from build123d import *

# Parameters (mm, degrees)
F1_DEPTH = 60
F2_SIZE  = 1


with BuildPart() as f1:
    # F0 (on Front) → F1 (new body)
    with BuildSketch(Plane.XZ):
        with BuildLine():
            Line((1.82927, 49.370132), (0, 50))
            Line((0, 50), (2.288286, 42.019797))
            ThreePointArc((2.288286, 42.019797), (1.404131, 39.441349), (-1.321078, 39.383352))
            Line((-1.321078, 39.383352), (-13.51647, 47.519061))
            Line((-13.51647, 47.519061), (-15.45085, 47.552826))
            Line((-15.45085, 47.552826), (-10.808542, 40.670321))
            ThreePointArc((-10.808542, 40.670321), (-10.852639, 37.944852), (-13.426545, 37.047558))
            Line((-13.426545, 37.047558), (-27.539125, 41.016494))
            Line((-27.539125, 41.016494), (-29.389263, 40.45085))
            Line((-29.389263, 40.45085), (-22.847355, 35.339751))
            ThreePointArc((-22.847355, 35.339751), (-22.047077, 32.734049), (-24.217728, 31.085291))
            Line((-24.217728, 31.085291), (-38.866057, 30.498946))
            Line((-38.866057, 30.498946), (-40.45085, 29.389263))
            Line((-40.45085, 29.389263), (-32.649709, 26.54988))
            ThreePointArc((-32.649709, 26.54988), (-31.083394, 24.319009), (-32.638311, 22.080179))
            Line((-32.638311, 22.080179), (-46.38851, 16.995949))
            Line((-46.38851, 16.995949), (-47.552826, 15.45085))
            Line((-47.552826, 15.45085), (-39.256083, 15.161121))
            ThreePointArc((-39.256083, 15.161121), (-37.077051, 13.523455), (-37.864029, 10.913705))
            Line((-37.864029, 10.913705), (-49.370132, 1.82927))
            Line((-49.370132, 1.82927), (-50, 0))
            Line((-50, 0), (-42.019797, 2.288286))
            ThreePointArc((-42.019797, 2.288286), (-39.441349, 1.404131), (-39.383352, -1.321078))
            Line((-39.383352, -1.321078), (-47.519061, -13.51647))
            Line((-47.519061, -13.51647), (-47.552826, -15.45085))
            Line((-47.552826, -15.45085), (-40.670321, -10.808542))
            ThreePointArc((-40.670321, -10.808542), (-37.944852, -10.852639), (-37.047558, -13.426545))
            Line((-37.047558, -13.426545), (-41.016494, -27.539125))
            Line((-41.016494, -27.539125), (-40.45085, -29.389263))
            Line((-40.45085, -29.389263), (-35.339751, -22.847355))
            ThreePointArc((-35.339751, -22.847355), (-32.734049, -22.047077), (-31.085291, -24.217728))
            Line((-31.085291, -24.217728), (-30.498946, -38.866057))
            Line((-30.498946, -38.866057), (-29.389263, -40.45085))
            Line((-29.389263, -40.45085), (-26.54988, -32.649709))
            ThreePointArc((-26.54988, -32.649709), (-24.319009, -31.083394), (-22.080179, -32.638311))
            Line((-22.080179, -32.638311), (-16.995949, -46.38851))
            Line((-16.995949, -46.38851), (-15.45085, -47.552826))
            Line((-15.45085, -47.552826), (-15.161121, -39.256083))
            ThreePointArc((-15.161121, -39.256083), (-13.523455, -37.077051), (-10.913705, -37.864029))
            Line((-10.913705, -37.864029), (-1.82927, -49.370132))
            Line((-1.82927, -49.370132), (0, -50))
            Line((0, -50), (-2.288286, -42.019797))
            ThreePointArc((-2.288286, -42.019797), (-1.404131, -39.441349), (1.321078, -39.383352))
            Line((1.321078, -39.383352), (13.51647, -47.519061))
            Line((13.51647, -47.519061), (15.45085, -47.552826))
            Line((15.45085, -47.552826), (10.808542, -40.670321))
            ThreePointArc((10.808542, -40.670321), (10.852639, -37.944852), (13.426545, -37.047558))
            Line((13.426545, -37.047558), (27.539125, -41.016494))
            Line((27.539125, -41.016494), (29.389263, -40.45085))
            Line((29.389263, -40.45085), (22.847355, -35.339751))
            ThreePointArc((22.847355, -35.339751), (22.047077, -32.734049), (24.217728, -31.085291))
            Line((24.217728, -31.085291), (38.866057, -30.498946))
            Line((38.866057, -30.498946), (40.45085, -29.389263))
            Line((40.45085, -29.389263), (32.649709, -26.54988))
            ThreePointArc((32.649709, -26.54988), (31.083394, -24.319009), (32.638311, -22.080179))
            Line((32.638311, -22.080179), (46.38851, -16.995949))
            Line((46.38851, -16.995949), (47.552826, -15.45085))
            Line((47.552826, -15.45085), (39.256083, -15.161121))
            ThreePointArc((39.256083, -15.161121), (37.077051, -13.523455), (37.864029, -10.913705))
            Line((37.864029, -10.913705), (49.370132, -1.82927))
            Line((49.370132, -1.82927), (50, 0))
            Line((50, 0), (42.019797, -2.288286))
            ThreePointArc((42.019797, -2.288286), (39.441349, -1.404131), (39.383352, 1.321078))
            Line((39.383352, 1.321078), (47.519061, 13.51647))
            Line((47.519061, 13.51647), (47.552826, 15.45085))
            Line((47.552826, 15.45085), (40.670321, 10.808542))
            ThreePointArc((40.670321, 10.808542), (37.944852, 10.852639), (37.047558, 13.426545))
            Line((37.047558, 13.426545), (41.016494, 27.539125))
            Line((41.016494, 27.539125), (40.45085, 29.389263))
            Line((40.45085, 29.389263), (35.339751, 22.847355))
            ThreePointArc((35.339751, 22.847355), (32.734049, 22.047077), (31.085291, 24.217728))
            Line((31.085291, 24.217728), (30.498946, 38.866057))
            Line((30.498946, 38.866057), (29.389263, 40.45085))
            Line((29.389263, 40.45085), (26.54988, 32.649709))
            ThreePointArc((26.54988, 32.649709), (24.319009, 31.083394), (22.080179, 32.638311))
            Line((22.080179, 32.638311), (16.995949, 46.38851))
            Line((16.995949, 46.38851), (15.45085, 47.552826))
            Line((15.45085, 47.552826), (15.161121, 39.256083))
            ThreePointArc((15.161121, 39.256083), (13.523455, 37.077051), (10.913705, 37.864029))
            Line((10.913705, 37.864029), (1.82927, 49.370132))
        make_face()
        with BuildLine():
            ThreePointArc((-4, -19.595918), (0, 20), (4, -19.595918))
            Line((4, -19.595918), (4, -23.595918))
            Line((4, -23.595918), (-4, -23.595918))
            Line((-4, -23.595918), (-4, -19.595918))
        make_face(mode=Mode.SUBTRACT)
    extrude(amount=F1_DEPTH)

    # F2
    f2_edges = [f1.edges().sort_by_distance(p)[0] for p in [
        (0, -60, 20),
        (0, 0, 20),
    ]]
    chamfer(f2_edges, length=F2_SIZE)


solid = f1.part
Work out the finished part from the listing and answer in its coordinate system (mm). A direction names the side the tool comes from. Coordinates: 2 decimals unless noted, no trailing zeros. Answer in a Markdown table with one row per item. Add a question column.
1. A tool of negligible diameter and unlimited length cuts with its end or side. For faces 1 (the flat face through (-31.439, -29.58, 30.796)), 2 (the flat face through (-4, -30, -22)), 3 (the flat face through (37.93, -29.58, 26.16)), 4 (the flat face through (26.16, -29.58, -37.93)), from which of +Z, -Z, +X, -X, +Y, -Y can it reach the whole face along a straight path? Write none if from no direction.
2. Flat-ended cylindrical pins translate along their axes: P1, Ø3, axis at x = -32, y = -36, coming from the +Z side; P2, Ø3, axis at x = -38.5, y = -41.5, coming from the -Z side; P3, Ø6, axis at y = -14.5, z = -0.5, coming from the -X side. Find the tip coordinate at first contact, or state that the pin passes through.
3. The mould has two halves that part along Z. Classify faces 5 (the flat face through (-39.004, -29.58, -20.384)), 6 (the cylindrical face through (13.56, -29.58, 37.09)), 7 (the flat face through (-1.128, -29.58, -46.066)), 8 (the cylindrical face through (-13.56, -29.58, -37.09)): pulls with the +Z half, pulls with the -Z half, needs draft (parallel to the pull), parting line crosses it, or undercut.
4. Consider L1, parallel to X at y = -31.5, z = -4.5; L2, parallel to Z at x = -6, y = -14; L3, parallel to Z at x = -7.5, y = -52.5. Determine where each line is inside the solid, lowest interval first.
Reported:
| question | item | result |
|---|---|---|
| 1 | face 1 | -X, +Y, -Y |
| 1 | face 2 | +Y, -Y |
| 1 | face 3 | +Z, +Y, -Y |
| 1 | face 4 | +X, +Y, -Y |
| 2 | P1 | stops at z = 30.83 |
| 2 | P2 | stops at z = -28.81 |
| 2 | P3 | stops at x = -50 |
| 3 | face 5 | undercut |
| 3 | face 6 | pulls with the +Z half |
| 3 | face 7 | undercut |
| 3 | face 8 | pulls with the -Z half |
| 4 | L1 | x = -41.5 to -19.49, 19.49 to 45.99 |
| 4 | L2 | z = -44.09 to -19.08, 19.08 to 42.5 |
| 4 | L3 | z = -42.19 to -18.54, 18.54 to 43.51 |
